Here's how the part is built. I have some questions about the finished solid (model axes, mm). Give positions to 0.01 mm unless a question says otherwise; leave off trailing zeros. Loops run counter-clockwise (first coordinate to the right, second up) from the corner with the lowest first, then second, coordinate; pieces in that order, holes last. Notation, with made-up numbers: (84.5, 32) - (91.5, 32) arc R4 cw to (91.5, 38) - close; hole circle Ø11 at (87.25, 7). An arc over 180 degrees is marked (long way). Use a Markdown table: item, result.
Solid Edge part; units mm, degrees
sketch "Sketch1" plane through (0, 0, 0) normal (0, 0, 1) x (1, 0, 0)
  line L0 (2.8868, 5) -> (5.7735, 0)
  line L1 (5.7735, 0) -> (2.8868, -5)
  line L2 (2.8868, -5) -> (-2.8868, -5)
  line L3 (-5.7735, 0) -> (-2.8868, -5)
  line L4 (-2.8868, 5) -> (-5.7735, 0)
  line L5 (-2.8868, 5) -> (2.8868, 5)
extrude "Protrusion1" add sketch "Sketch1" along normal blind 5
hole "Hole_1" at (0, 0, 5) direction (0, 0, -1) diameter 4.917 end up to next
sketch "Sketch2" plane through (0, 0, 0) normal (1, 0, 0) x (0, 1, 0)
  line L0 (-4.8586, 4.8586) -> (-3.7954, 5.9218)
revolve "RevolvedCutout1" cut sketch "Sketch2" angle 360 about axis through (0, 0, -57) along (0, 0, 1) material side at (0, -4.3624, 5.4256)
mirror "Mirror1" about plane through (0, 0, 2.5) normal (0, 0, 1) of "RevolvedCutout1"
(1) Suppose I cut it at B-B on x = 0. Write out the boundary of the cut face in (y, z), plus the area to 3 significant figures.
A:
| item | result |
|---|---|
| outline | (-5, 0.28) - (-4.72, 0) - (-2.46, 0) - (-2.46, 5) - (-4.72, 5) - (-5, 4.72) - close; (2.46, 0) - (4.72, 0) - (5, 0.28) - (5, 4.72) - (4.72, 5) - (2.46, 5) - close |
| area | 25.3 mm2 |
(2) We'd pull the mould along X, two halves only. Please class faces 1 (the face through (4.35, -2.465, 2.469)), 2 (the face through (-4.31, 2.535, 2.469)), 3 (the face through (0.738, -2.345, 2.535)), 4 (the face through (-2, -2, 0)): pulls with the +X half, pulls with the -X half, needs draft (parallel to the pull), parting line crosses it, or undercut.
A:
| item | result |
|---|---|
| face 1 | pulls with the +X half |
| face 2 | pulls with the -X half |
| face 3 | undercut |
| face 4 | needs draft |
(3) Suppose I cut it at C-C on z = 4.3. Write out the boundary of the cut face in (x, y).
A:
| item | result |
|---|---|
| outline | (-5.37, -0.69) - (-3.29, -4.31) arc R5.42 ccw to (-2.08, -5) - (2.08, -5) arc R5.42 ccw to (3.29, -4.31) - (5.37, -0.69) arc R5.42 ccw to (5.37, 0.69) - (3.29, 4.31) arc R5.42 ccw to (2.08, 5) - (-2.08, 5) arc R5.42 ccw to (-3.29, 4.31) - (-5.37, 0.69) arc R5.42 ccw to start; hole circle Ø4.92 at (0, 0) |
(4) Will these pins go through, and if not, where does the flat tip stop? pin 1 (3 mm diameter, centred on y = 2.5, z = 3.5, fed in from +X); pin 2 (4.5 mm diameter, centred on x = 0, y = 0, fed in from -Z).
A:
| item | result |
|---|---|
| pin 1 | x = 5.2 |
| pin 2 | through |
(5) If I drill on line 1 (Y direction, x = 0, z = 2.4); line 2 (Y direction, x = -0.5, z = 0.8); line 3 (X direction, y = 1, z = 1.55), over which ranges is the centre line in solid material (lowest first)?
A:
| item | result |
|---|---|
| line 1 | -5 to -2.46, 2.46 to 5 |
| line 2 | -5 to -2.41, 2.41 to 5 |
| line 3 | -5.2 to -2.25, 2.25 to 5.2 |
(6) Suppose I cut it at A-A on z = 1.95. Write out the boundary of the cut face in (x, y).
A:
| item | result |
|---|---|
| outline | (-5.77, 0) - (-2.89, -5) - (2.89, -5) - (5.77, 0) - (2.89, 5) - (-2.89, 5) - close; hole circle Ø4.92 at (0, 0) |
